from build123d import *

# Parameters (mm, degrees)
SKETCH_1_R      = 10
EXTRUDE_1_DEPTH = 2
SKETCH_2_W      = 13.356704287
SKETCH_2_H      = 30
EXTRUDE_2_DEPTH = 2


with BuildPart() as part:
    # 草图1 → 凸台-拉伸1 (new body)
    with BuildSketch(Plane(origin=(0, 0, 0), x_dir=(1, 0, 0), z_dir=(0, 1, 0))):
        with BuildLine():
            Line((0, 15), (50, 15))
            ThreePointArc((50, 15), (65, 0), (50, -15))
            Line((50, -15), (0, -15))
            ThreePointArc((0, -15), (-15, 0), (0, 15))
        make_face()
        with Locations(Location((0, 0, 0), (0, 0, 270))):
            Circle(SKETCH_1_R, mode=Mode.SUBTRACT)
        with Locations(Location((50, 0, 0), (0, 0, 270))):
            Circle(SKETCH_1_R, mode=Mode.SUBTRACT)
    extrude_1 = extrude(amount=EXTRUDE_1_DEPTH)

    # 草图2 → 凸台-拉伸2 (add)
    with BuildSketch(Plane(origin=(0, 2, 0), x_dir=(1, 0, 0), z_dir=(0, 1, 0))):
        with Locations((20.097558378, 0)):
            Rectangle(SKETCH_2_W, SKETCH_2_H)
    extrude_2 = extrude(amount=EXTRUDE_2_DEPTH)

    # 镜向1: 凸台-拉伸1, 凸台-拉伸2 across plane
    add(extrude_1.mirror(Plane.ZX.offset(4)))
    add(extrude_2.mirror(Plane.ZX.offset(4)))


solid = part.part
Can you work these out from the model? Positions are in its coordinate system, mm. A direction names the side the tool comes from. Give positions to 0.01 mm unless a question says otherwise; leave off trailing zeros. Order: outer loops, then holes, each group sorted by start corner. A loop starts at its lowest first (then second) coordinate and runs counter-clockwise, first axis right, second up. Notation, with made-up numbers: M 33,-30.75 L 37,-30.75 A16 ccw 37,-0.75 Z; hole C 43.5,1.25 d6. An arc over 180 degrees is marked long. Use a Markdown table: item, result. Add a question column.
Item 1: Will these pins go through, and if not, where does the flat tip stop? pin 1 (1.2 mm diameter, centred on y = 3.5, z = 2.5, fed in from -X); pin 2 (3 mm diameter, centred on y = 4, z = 11, fed in from +X).
Item 2: Suppose I cut it at B-B (z = 0). List the corners of the cut face in (x, y) for me, then the cut area to 3 significant figures.
Item 3: Suppose I cut it at D-D (y = 7). List the corners of the cut face in (x, z) for me, then the cut area to 3 significant figures.
Item 4: Suppose I cut it at A-A (x = 8). List the corners of the cut face in (y, z) for me, then the cut area to 3 significant figures.
Item 5: We'd pull the mould along Y, two halves only. Please class faces 4 (the flat face through (26.776, 4, 0)), 5 (the cylindrical face through (65, 7, 0)), 6 (the flat face through (26, 8, 0)): +Y half, -Y half, draft (parallel to the pull), parting line (faces both ways), or undercut.
Item 6: For faces 1 (the flat face through (13.419, 4, 0)), 2 (the flat face through (26, 0, 0)), 3 (the flat face through (38, 2, 0)), which set-ups out of +Z, -Z, +X, -X, +Y, -Y let a thin tool reach every point of the face, with its end or its side?
Item 7: If I drill on L1, parallel to X at y = 6.75, z = 0; L2, parallel to X at y = 6.5, z = -3.5; L3, parallel to Y at x = 9, z = 10.5, over which ranges is the centre line in solid material (lowest first)? Write a range as [from, to].
Item 8: Suppose I cut it at C-C (z = 12). List the corners of the cut face in (x, y) for me.
Answer sheet:
| question | item | result |
|---|---|---|
| 1 | pin 1 | stops at x = 13.42 |
| 1 | pin 2 | stops at x = 26.78 |
| 2 | outline | M -15,0 L -10,0 L -10,2 L -15,2 Z; M -15,6 L -10,6 L -10,8 L -15,8 Z; M 10,0 L 40,0 L 40,2 L 26.78,2 L 26.78,6 L 40,6 L 40,8 L 10,8 L 10,6 L 13.42,6 L 13.42,2 L 10,2 Z; M 60,0 L 65,0 L 65,2 L 60,2 Z; M 60,6 L 65,6 L 65,8 L 60,8 Z |
| 2 | area | 213 mm² |
| 3 | outline | M 0,-15 L 50,-15 A15 ccw 50,15 L 0,15 A15 ccw Z; hole C 0,0 d20; hole C 50,0 d20 |
| 3 | area | 1,580 mm² |
| 4 | outline | M 0,-15 L 2,-15 L 2,-6 L 0,-6 Z; M 0,6 L 2,6 L 2,15 L 0,15 Z; M 6,-15 L 8,-15 L 8,-6 L 6,-6 Z; M 6,6 L 8,6 L 8,15 L 6,15 Z |
| 4 | area | 72.0 mm² |
| 5 | face 4 | undercut |
| 5 | face 5 | draft |
| 5 | face 6 | +Y half |
| 6 | face 1 | +Z, -Z, -X |
| 6 | face 2 | +Z, -Z, +X, -X, -Y |
| 6 | face 3 | +Z, -Z, +X |
| 7 | L1 | x = [-15, -10], [10, 40], [60, 65] |
| 7 | L2 | x = [-14.59, -9.37], [9.37, 40.63], [59.37, 64.59] |
| 7 | L3 | y = [0, 2], [6, 8] |
| 8 | outline | M -9,0 L 59,0 L 59,2 L 26.78,2 L 26.78,6 L 59,6 L 59,8 L -9,8 L -9,6 L 13.42,6 L 13.42,2 L -9,2 Z |
